```python
from build123d import *

# Parameters (mm, degrees)
SKETCH1_R           = 55
BOSS_EXTRUDE1_DEPTH = 3
SKETCH2_R           = 43
BOSS_EXTRUDE2_DEPTH = 50
SKETCH3_R           = 40
CUT_EXTRUDE1_DEPTH  = 66
SKETCH10_R          = 4.5
CUT_EXTRUDE2_DEPTH  = 9
BOSS_EXTRUDE4_DEPTH = 5
SKETCH17_W          = 10.5
SKETCH17_H          = 3
BOSS_EXTRUDE7_DEPTH = 10.5
CUT_EXTRUDE6_DEPTH  = 3
SKETCH19_W          = 29.5
SKETCH19_H          = 3
BOSS_EXTRUDE8_DEPTH = 10.5
CUT_EXTRUDE7_DEPTH  = 3
SKETCH21_R          = 1.5
CUT_EXTRUDE8_DEPTH  = 8
CIRPATTERN1_COUNT   = 3
SKETCH23_R          = 1
CUT_EXTRUDE9_DEPTH  = 9
SKETCH24_R          = 1
CUT_EXTRUDE10_DEPTH = 9


with BuildPart() as part:
    # Sketch1 → Boss-Extrude1 (new body)
    with BuildSketch(Plane(origin=(0, 0, 0), x_dir=(1, 0, 0), z_dir=(0, 1, 0))):
        with Locations(Location((0, 0, 0), (0, 0, 270))):
            Circle(SKETCH1_R)
    extrude(amount=BOSS_EXTRUDE1_DEPTH)

    # Sketch2 → Boss-Extrude2 (add)
    with BuildSketch(Plane(origin=(0, 3, 0), x_dir=(1, 0, 0), z_dir=(0, 1, 0))):
        with Locations(Location((0, 0, 0), (0, 0, 270))):
            Circle(SKETCH2_R)
    extrude(amount=BOSS_EXTRUDE2_DEPTH)

    # Sketch3 → Cut-Extrude1 (cut)
    with BuildSketch(Plane(origin=(0, 53, 0), x_dir=(1, 0, 0), z_dir=(0, 1, 0))):
        with Locations(Location((0, 0, 0), (0, 0, 270))):
            Circle(SKETCH3_R)
    extrude(amount=-CUT_EXTRUDE1_DEPTH, mode=Mode.SUBTRACT)

    # Sketch10 → Cut-Extrude2 (cut)
    with BuildSketch(Plane(origin=(-39, 0, 0), x_dir=(0, 0, -1), z_dir=(1, 0, 0))):
        with Locations((0, 13)):
            Circle(SKETCH10_R)
    extrude(amount=-CUT_EXTRUDE2_DEPTH, mode=Mode.SUBTRACT)

    # Sketch12 → Boss-Extrude4 (add)
    with BuildSketch(Plane(origin=(0, 35, 0), x_dir=(1, 0, 0), z_dir=(0, 1, 0))):
        with BuildLine():
            Line((-11, 10), (-39.761790704, 10))
            ThreePointArc((-39.761790704, 10), (-41, 0), (-39.761790704, -10))
            Line((-39.761790704, -10), (-11, -10))
            Line((-11, -10), (-11, 10))
        make_face()
        with BuildLine():
            Line((30, 10), (39.761790704, 10))
            ThreePointArc((39.761790704, 10), (41, 0), (39.761790704, -10))
            Line((39.761790704, -10), (30, -10))
            Line((30, -10), (30, 10))
        make_face()
    extrude(amount=-BOSS_EXTRUDE4_DEPTH)

    # Sketch17 → Boss-Extrude7 (add)
    with BuildSketch(Plane.XZ.offset(-30)):
        with Locations((35.25, 0)):
            Rectangle(SKETCH17_W, SKETCH17_H)
    extrude(amount=BOSS_EXTRUDE7_DEPTH)

    # Sketch18 → Cut-Extrude6 (cut)
    with BuildSketch(Plane.XY.offset(1.5)):
        Polygon((30, 30), (39.971865105, 19.5), (30, 19.5), align=None)
    extrude(amount=-CUT_EXTRUDE6_DEPTH, mode=Mode.SUBTRACT)

    # Sketch19 → Boss-Extrude8 (add)
    with BuildSketch(Plane.XZ.offset(-30)):
        with Locations((-25.75, 0)):
            Rectangle(SKETCH19_W, SKETCH19_H)
    extrude(amount=BOSS_EXTRUDE8_DEPTH)

    # Sketch20 → Cut-Extrude7 (cut)
    with BuildSketch(Plane.XY.offset(1.5)):
        Polygon((-39.971865105, 19.5), (-11, 30), (-11, 19.5), align=None)
    extrude(amount=-CUT_EXTRUDE7_DEPTH, mode=Mode.SUBTRACT)

    # Sketch21 → Cut-Extrude8 (cut)
    with BuildSketch(Plane(origin=(0, 3, 0), x_dir=(1, 0, 0), z_dir=(0, 1, 0))):
        with Locations(Location((49, 0, 0), (0, 0, 270))):
            Circle(SKETCH21_R)
    cut_extrude8 = extrude(amount=-CUT_EXTRUDE8_DEPTH, mode=Mode.SUBTRACT)

    # CirPattern1: Cut-Extrude8 ×3 about axis
    cirpattern1_axis = Axis((0, 0, 0), (0, 1, 0))
    for i in range(1, CIRPATTERN1_COUNT):
        add(cut_extrude8.rotate(cirpattern1_axis, i * 360 / CIRPATTERN1_COUNT), mode=Mode.SUBTRACT)

    # Sketch23 → Cut-Extrude9 (cut)
    with BuildSketch(Plane(origin=(0, 35, 0), x_dir=(1, 0, 0), z_dir=(0, 1, 0))):
        with Locations(Location((-14.5, 5, 0), (0, 0, 270))):
            Circle(SKETCH23_R)
        with Locations(Location((-14.5, -5, 0), (0, 0, 270))):
            Circle(SKETCH23_R)
    extrude(amount=-CUT_EXTRUDE9_DEPTH, mode=Mode.SUBTRACT)

    # Sketch24 → Cut-Extrude10 (cut)
    with BuildSketch(Plane(origin=(0, 35, 0), x_dir=(1, 0, 0), z_dir=(0, 1, 0))):
        with Locations(Location((33.5, 5, 0), (0, 0, 270))):
            Circle(SKETCH24_R)
        with Locations(Location((33.5, -5, 0), (0, 0, 270))):
            Circle(SKETCH24_R)
    extrude(amount=-CUT_EXTRUDE10_DEPTH, mode=Mode.SUBTRACT)


solid = part.part
```
Verification items for the finished model (mm, model axes). A direction names the side the tool comes from. Coordinates: 2 decimals unless noted, no trailing zeros. Order: outer loops, then holes, each group sorted by start corner. A loop starts at its lowest first (then second) coordinate and runs counter-clockwise, first axis right, second up. Notation, with made-up numbers: (-28.5, -9) -> (1.5, -9) arc R17 ccw to (1.5, -5) -> close; hole circle Ø2 at (77, 4). An arc over 180 degrees is marked (long way). Put each result on its own line as item: value. Start each with the question number.
1) Release check for a two-part mould opening along Y. For faces 1 (the cylindrical face through (-41.351, 13.198, 4.496)), 2 (the flat face through (-26, 30, 6)), 3 (the flat face through (-25, 33, 10)) record: pulls with the +Y half, pulls with the -Y half, needs draft (parallel to the pull), parting line crosses it, or undercut.
2) Material ranges on L1, parallel to X at y = 1.3, z = 0; L2, parallel to Z at x = -1.5, y = 21; L3, parallel to Z at x = -14, y = 32, recorded low to high.
3) Cross-section at B-B (z = 0). State how many separate pieces and enclosed holes the cut face has, plus the area to 3 significant figures.
4) Cross-section at C-C (x = -33). Enter the section's corners in (y, z), plus the area to 3 significant figures.
5) Cross-section at D-D (y = 23.5). Enter the section's corners in (x, z).
6) Cross-section at A-A (x = 49). Enter the section's corners in (y, z).
7) Tool access check on faces 4 (the flat face through (29, 0, 28)), 5 (the flat face through (29, 3, 32)), 6 (the flat face through (34.92, 24.82, 0.02)), 7 (the flat face through (34, 33, 10)), 8 (the flat face through (-38, 53, 13)). Record the directions out of +Z, -Z, +X, -X, +Y, -Y that give a thin tool (end or side, any length) a straight path to the whole face; none if there is none.
8) Go/stop test with flat-tipped pins: pin 1 (8 mm diameter, centred on x = -12, y = 40, fed in from +Z); pin 2 (5 mm diameter, centred on y = 39, z = 16, fed in from -X); pin 3 (7 mm diameter, centred on x = 33, z = -5.5, fed in from -Y); pin 4 (1.8 mm diameter, centred on x = -14.5, z = 5, fed in from -Y). Record where each tip stops, or that it passes through.
Geometry check:
1. face 1: undercut
1. face 2: pulls with the -Y half
1. face 3: needs draft
2. L1: x = -55 to -40, 40 to 47.5, 50.5 to 55
2. L2: z = -42.97 to -39.97, 39.97 to 42.97
2. L3: z = -40.66 to -37.47, -10 to -5.87, -4.13 to 4.13, 5.87 to 10, 37.47 to 40.66
3. separate pieces: 4
3. enclosed holes: 0
3. area: 754 mm^2
4. outline: (0, -44) -> (3, -44) -> (3, -27.57) -> (53, -27.57) -> (53, -22.61) -> (0, -22.61) -> close; (0, 22.61) -> (53, 22.61) -> (53, 27.57) -> (3, 27.57) -> (3, 44) -> (0, 44) -> close; (22.03, -1.5) -> (30, -1.5) -> (30, -10) -> (35, -10) -> (35, 10) -> (30, 10) -> (30, 1.5) -> (22.03, 1.5) -> close
4. area: 749 mm^2
5. outline: circle Ø86 at (0, 0); hole (-39.97, -1.5) arc R40 ccw to (39.97, -1.5) -> (36.17, -1.5) -> (36.17, 1.5) -> (39.97, 1.5) arc R40 ccw to (-39.97, 1.5) -> (-28.93, 1.5) -> (-28.93, -1.5) -> close
6. outline: (0, -24.98) -> (3, -24.98) -> (3, -1.5) -> (0, -1.5) -> close; (0, 1.5) -> (3, 1.5) -> (3, 24.98) -> (0, 24.98) -> close
7. face 4: +Z, -Z, +X, -X, -Y
7. face 5: +Y
7. face 6: -Y
7. face 7: +Y, -Y
7. face 8: +Z, -Z, +X, -X, +Y
8. pin 1: stops at z = 42.25
8. pin 2: stops at x = -40.83
8. pin 3: stops at y = 30
8. pin 4: passes through
